```python
from build123d import *

# Parameters (mm, degrees)
SKETCH1_R           = 1.5
SKETCH1_R_2         = 10
BOSS_EXTRUDE1_DEPTH = 2
SKETCH2_W           = 2
SKETCH2_H           = 38
BOSS_EXTRUDE2_DEPTH = 43
FILLET1_R           = 2
CUT_EXTRUDE1_DEPTH  = 77.5


with BuildPart() as part:
    # Sketch1 → Boss-Extrude1 (new body)
    with BuildSketch(Plane(origin=(0, 0, 0), x_dir=(1, 0, 0), z_dir=(0, 1, 0))):
        with BuildLine():
            Line((0, 0), (61.387482194, 0))
            Line((61.387482194, 0), (61.387482194, 38))
            Line((61.387482194, 38), (0, 38))
            ThreePointArc((0, 38), (-15.112517806, 19), (0, 0))
        make_face()
        with Locations((-9.612517806, 19)):
            Circle(SKETCH1_R, mode=Mode.SUBTRACT)
        with Locations((11.387482194, 31.124355653)):
            Circle(SKETCH1_R, mode=Mode.SUBTRACT)
        with Locations((11.387482194, 6.875644347)):
            Circle(SKETCH1_R, mode=Mode.SUBTRACT)
        with Locations((4.387482194, 19)):
            Circle(SKETCH1_R_2, mode=Mode.SUBTRACT)
    extrude(amount=BOSS_EXTRUDE1_DEPTH)

    # Sketch2 → Boss-Extrude2 (add)
    with BuildSketch(Plane(origin=(0, 2, 0), x_dir=(1, 0, 0), z_dir=(0, 1, 0))):
        with Locations((60.387482194, 19)):
            Rectangle(SKETCH2_W, SKETCH2_H)
    extrude(amount=BOSS_EXTRUDE2_DEPTH)

    # Fillet1
    fillet1_edges = [part.edges().sort_by_distance(p)[0] for p in [
        (61.387482194, 0, -19),
        (59.387482194, 2, -19),
        (60.387482194, 45, -38),
        (60.387482194, 45, 0),
    ]]
    fillet(fillet1_edges, radius=FILLET1_R)

    # Sketch3 → Cut-Extrude1 (cut, through all)
    with BuildSketch(Plane(origin=(61.387482194, 0, 0), x_dir=(0, 0, -1), z_dir=(1, 0, 0))):
        with BuildLine():
            Line((10, 39), (10, 31))
            ThreePointArc((10, 31), (6, 27), (2, 31))
            Line((2, 31), (2, 39))
            ThreePointArc((2, 39), (6, 43), (10, 39))
        make_face()
        with BuildLine():
            Line((36, 39), (36, 31))
            ThreePointArc((36, 31), (32, 27), (28, 31))
            Line((28, 31), (28, 39))
            ThreePointArc((28, 39), (32, 43), (36, 39))
        make_face()
    extrude(amount=-CUT_EXTRUDE1_DEPTH, mode=Mode.SUBTRACT)


solid = part.part
```
Geometry: final body of the model. Coordinates: model frame, mm. A direction names the side the tool comes from. Round coordinates to 2 decimals unless told otherwise and drop trailing zeros. Loops run counter-clockwise (first coordinate to the right, second up) from the corner with the lowest first, then second, coordinate; pieces in that order, holes last. Notation, with made-up numbers: (-14, 37) -> (32, 37) arc R25 ccw to (32, 54) -> close; hole circle Ø3 at (21.5, 51). An arc over 180 degrees is marked (long way). Use one line per item in the form item = value. Start each with the question number.
1) Section D-D on x = 34. Output: boundary loops of the cut face in (y, z), then the cut area to 3 significant figures.
2) First-contact query: P1, Ø5, axis at x = 11.39, z = -6.88, coming from the +Y side; P2, Ø6, axis at y = 8, z = -18, coming from the -X side; P3, Ø8, axis at x = 1.5, z = -22.5, coming from the -Y side. Flat tips, straight axial feed; report the tip coordinate or a pass-through.
3) Section C-C on z = -34. Output: boundary loops of the cut face in (x, y), then the cut area to 3 significant figures.
4) Draft query along Y for faces 1 (the flat face through (60, 45, -19)), 2 (the flat face through (61.387, 23, -19)), 3 (the cylindrical face through (60, 27, -6)). Return one class per face: released by +Y, released by -Y, zero draft, split by the parting line, or undercut.
5) Access query for faces 4 (the flat face through (60, 35, -2)), 5 (the cylindrical face through (60.817, 0.601, -19.266)), 6 (the flat face through (29, 2, -19)). Directions: +Z, -Z, +X, -X, +Y, -Y. A direction counts if a zero-diameter tool reaches every point of the face in a straight line with its end or side. Return the directions, or none.
6) Line query: L1, parallel to X at y = 33, z = -13; L2, parallel to Y at x = -8, z = -24.5. Output: solid intervals per line, ascending.
7) Section B-B on y = 40. Output: boundary loops of the cut face in (x, z), then the cut area to 3 significant figures.
8) Section A-A on z = -19. Output: boundary loops of the cut face in (x, y), then the cut area to 3 significant figures.
Response:
q1.outline = (0, -38) -> (2, -38) -> (2, 0) -> (0, 0) -> close
q1.area = 76.0 mm^2
q2.P1 = 2
q2.P2 = 59.39
q2.P3 = through
q3.outline = (-8.07, 0) -> (59.39, 0) arc R2 ccw to (61.39, 2) -> (61.39, 27.54) -> (59.39, 27.54) -> (59.39, 4) arc R2 cw to (57.39, 2) -> (-8.07, 2) -> close; (59.39, 42.46) -> (61.39, 42.46) -> (61.39, 45) -> (59.39, 45) -> close
q3.area = 195 mm^2
q4.face_1 = released by +Y
q4.face_2 = zero draft
q4.face_3 = undercut
q5.face_4 = +X, -X
q5.face_5 = +Z, -Z, +X, -Y
q5.face_6 = +Z, -Z, -X, +Y
q6.L1 = 59.39 to 61.39
q6.L2 = 0 to 2
q7.outline = (59.39, -38) -> (61.39, -38) -> (61.39, -35.87) -> (59.39, -35.87) -> close; (59.39, -28.13) -> (61.39, -28.13) -> (61.39, -9.87) -> (59.39, -9.87) -> close; (59.39, -2.13) -> (61.39, -2.13) -> (61.39, 0) -> (59.39, 0) -> close
q7.area = 45.0 mm^2
q8.outline = (-15.11, 0) -> (-11.11, 0) -> (-11.11, 2) -> (-15.11, 2) -> close; (-8.11, 0) -> (-5.61, 0) -> (-5.61, 2) -> (-8.11, 2) -> close; (14.39, 0) -> (59.39, 0) arc R2 ccw to (61.39, 2) -> (61.39, 45) -> (59.39, 45) -> (59.39, 4) arc R2 cw to (57.39, 2) -> (14.39, 2) -> close
q8.area = 193 mm^2
